from build123d import *

# Parameters (mm, degrees)
EXTRUDE_1_DEPTH          = 12
CUT_EXTRUDE_1_DEPTH      = 10
CUT_EXTRUDE_1_DEPTH_BACK = 10
SKETCH_2_W               = 2.506204129
SKETCH_2_H               = 10.984391515
EXTRUDE_START            = -1.5
EXTRUDE_2_DEPTH          = 1.5
FILLET_1_R               = 0.4
EXTRUDE_3_DEPTH          = 1.5
EXTRUDE_4_REACH          = 26.208


with BuildPart() as part:
    # 草图1 → 凸台-拉伸1 (new, symmetric)
    with BuildSketch(Plane(origin=(0, 0, 0), x_dir=(0, 0, -1), z_dir=(1, 0, 0))):
        with BuildLine():
            ThreePointArc((0.424459717, 1.438691749), (-1.23881175, -0.84578097), (1.494480371, -0.128562902))
            Line((1.494480371, -0.128562902), (0.897098533, 0.285679978))
            Line((0.897098533, 0.285679978), (0.611565164, 0.285679978))
            ThreePointArc((0.611565164, 0.285679978), (0.658950486, 0.146319025), (0.675, 0))
            ThreePointArc((0.675, 0), (-0.609153227, -0.290787458), (0.424459717, 0.524841832))
            Line((0.424459717, 0.524841832), (0.424459717, 1.438691749))
        make_face()
        with BuildLine():
            Line((8.48773274, -4.977898486), (8.91741162, -4.358256311))
            Line((8.91741162, -4.358256311), (0.854750449, 1.232640122))
            ThreePointArc((0.854750449, 1.232640122), (1.328932969, 0.695655923), (1.5, 0))
            ThreePointArc((1.5, 0), (1.498619458, -0.064340668), (1.494480371, -0.128562902))
            Line((1.494480371, -0.128562902), (8.48773274, -4.977898486))
        make_face()
        with BuildLine():
            ThreePointArc((1.5, 0), (1.328932969, 0.695655923), (0.854750449, 1.232640122))
            ThreePointArc((0.854750449, 1.232640122), (0.647849504, 1.352882485), (0.424459717, 1.438691749))
            Line((0.424459717, 1.438691749), (0.424459717, 0.524841832))
            ThreePointArc((0.424459717, 0.524841832), (0.531635671, 0.415918878), (0.611565164, 0.285679978))
            Line((0.611565164, 0.285679978), (0.897098533, 0.285679978))
            Line((0.897098533, 0.285679978), (1.494480371, -0.128562902))
            ThreePointArc((1.494480371, -0.128562902), (1.498619458, -0.064340668), (1.5, 0))
        make_face()
    extrude(amount=EXTRUDE_1_DEPTH, both=True)

    # 草图2 → 切除-拉伸1 (cut, two sides: drawn at the far end of the back side and taken through both)
    with BuildSketch(Plane(origin=(0, 0, 0), x_dir=(1, 0, 0), z_dir=(0, 1, 0)).offset(-CUT_EXTRUDE_1_DEPTH_BACK)):
        with Locations((-11.255680748, 7.657884592)):
            Rectangle(SKETCH_2_W, SKETCH_2_H)
        with Locations((11.255680748, 7.657884592)):
            Rectangle(SKETCH_2_W, SKETCH_2_H)
    extrude(amount=CUT_EXTRUDE_1_DEPTH + CUT_EXTRUDE_1_DEPTH_BACK, mode=Mode.SUBTRACT)

    # 草图3 → 凸台-拉伸2 (add)
    with BuildSketch(Plane.ZY.offset(12).offset(EXTRUDE_START)):
        with BuildLine():
            Line((1.209536672, 0.887142063), (4.315061937, -3.346956229))
            Line((4.315061937, -3.346956229), (2.791074167, -3.281580786))
            Line((2.791074167, -3.281580786), (-0.41583993, -1.441206839))
            ThreePointArc((-0.41583993, -1.441206839), (1.229955601, -0.858608886), (1.209536672, 0.887142063))
        make_face()
    extrude(amount=EXTRUDE_2_DEPTH)

    # 圆角1
    # the kernel refuses this fillet: 0.4 mm, written as the material it takes off along each edge
    with BuildSketch(Plane(origin=(0, -4.977898486, -8.48773274), x_dir=(0, 0.5698336328652603, 0.8217600810793743), z_dir=(-1, 0, 0)), Plane(origin=(0, -4.358256311, -8.91741162), x_dir=(0, 0.5698336328652598, 0.8217600810793746), z_dir=(1, 0, 0))) as fillet_1_piece_1:
        with BuildLine():
            CenterArc((FILLET_1_R, FILLET_1_R), FILLET_1_R, 180, 90)
            Line((0, FILLET_1_R), (0, 0))
            Line((0, 0), (FILLET_1_R, 0))
        make_face()
    extrude(amount=11.002578683, mode=Mode.SUBTRACT)
    with BuildSketch(Plane(origin=(0, -4.358256311, -8.91741162), x_dir=(0, 0.5698336328652598, 0.8217600810793746), z_dir=(-1, 0, 0)), Plane(origin=(0, -4.977898486, -8.48773274), x_dir=(0, 0.5698336328652603, 0.8217600810793743), z_dir=(1, 0, 0))) as fillet_1_piece_2:
        with BuildLine():
            CenterArc((FILLET_1_R, -FILLET_1_R), FILLET_1_R, 90, 90)
            Line((0, -FILLET_1_R), (0, 0))
            Line((0, 0), (FILLET_1_R, 0))
        make_face()
    extrude(amount=11.002578683, mode=Mode.SUBTRACT)

    # 草图4 → 凸台-拉伸3 (add)
    with BuildSketch(Plane(origin=(12, 0, 0), x_dir=(0, 0, -1), z_dir=(1, 0, 0))):
        with BuildLine():
            Line((-1.361590085, -0.629342864), (-0.064760058, -4.70678049))
            Line((-0.064760058, -4.70678049), (1.358347945, -5.014160577))
            Line((1.358347945, -5.014160577), (6.052641572, -4.70678049))
            Line((6.052641572, -4.70678049), (2.165688834, -0.593999427))
            Line((2.165688834, -0.593999427), (1.494480371, -0.128562902))
            ThreePointArc((1.494480371, -0.128562902), (0.259056171, -1.477460626), (-1.361590085, -0.629342864))
        make_face()
    extrude(amount=-EXTRUDE_3_DEPTH)

    # 凸台-拉伸4: up to this face of the body (flat: up to its plane)
    extrude_4_end = Plane(part.part.faces().sort_by_distance((12, -3.083366952, -2.010931635))[0])
    # 草图5 → 凸台-拉伸4 (add, up to the picked face)
    with BuildSketch(Plane(origin=(10.002578683, 0, 0), x_dir=(0, 0, -1), z_dir=(1, 0, 0)), mode=Mode.PRIVATE) as extrude_4_sk1:
        Polygon((6.052641572, -4.70678049), (2.165688834, -0.593999427), (2.165688834, 0.323595257), (7.146064321, -3.129949789), align=None)
    extrude_4_tool1 = split(extrude(extrude_4_sk1.sketch, amount=EXTRUDE_4_REACH, mode=Mode.PRIVATE), bisect_by=extrude_4_end, keep=Keep.BOTH, mode=Mode.PRIVATE)
    add(extrude_4_tool1.solids().sort_by(Axis((10.002579, -2.305975, -4.731819), (1, 0, 0)))[0])


solid = part.part
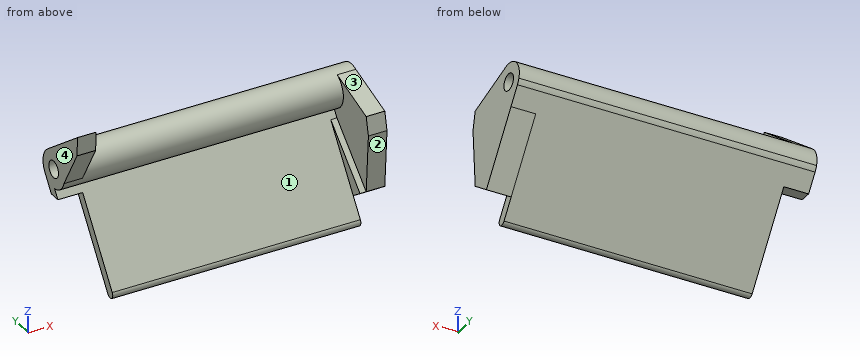
For this review, take the finished solid that the model builds, in its own axes (mm). Face numbers are marked on the shaded views. Round coordinates to 2 decimals unless told otherwise and drop trailing zeros. Write each loop counter-clockwise with the first axis right and the second up, starting at its lowest first coordinate (ties: lowest second). Pieces come first, ordered by that corner, then holes. Notation, with made-up numbers: (37.25, 0) -> (56.25, 0) arc R21 cw to (56.25, 23) -> close; hole circle Ø8 at (-11.5, -20.75). An arc over 180 degrees is marked (long way). Use CSV: the item, a comma, the result in double quotes.
(1) Consider section D-D, the plane z = -7.5. Give the boundary of the cut face in (x, y), plus the area to 3 significant figures.
Computed values:
outline,"(-10, -4.29) -> (10, -4.29) -> (10, -3.38) -> (-10, -3.38) -> close"
area,"18.4 mm²"
(2) To check wall thickness, follow L1, parallel to Y at x = 4, z = 0 (3 decimals); L2, parallel to Z at x = -9.75, y = -0.25; L3, parallel to X at y = -1.5, z = 0.5. State the ranges of each line that lie inside material, in increasing order. Write a range as [from, to].
Computed values:
L1,"[-1.5, -0.675], [0.675, 1.5]"
L2,"[-2.99, -1.67], [-1.48, -0.63], [0.63, 1.48]"
L3,"[-12, -10.5], [10.5, 12]"
(3) Consider section A-A, the plane y = -2. Give the boundary of the cut face in (x, z).
Computed values:
outline,"(-12, 0.56) -> (-10.5, 0.56) -> (-10.5, 3.33) -> (-12, 3.33) -> close; (-10, -5.52) -> (12, -5.52) -> (12, 0.93) -> (10.5, 0.93) -> (10.5, -3.49) -> (10, -3.49) -> (10, -4.19) -> (-10, -4.19) -> close"
(4) Consider section C-C, the plane z = 1.75. Give the boundary of the cut face in (x, y).
Computed values:
outline,"(-12, -2.68) -> (-10.5, -2.68) -> (-10.5, 0.15) -> (-12, 0.15) -> close"
(5) Clearance check with flat-ended pins moving along their axes: P1, Ø0.8, axis at y = -4, z = -7.5, coming from the +X side; P2, Ø3, axis at x = -4, z = -3, coming from the +Y side; P3, Ø1, axis at y = -3, z = -6, coming from the -X side; P4, Ø1.1, axis at y = 0, z = 0, coming from the -X side. State where each tip first meets the part, or that it passes through.
Computed values:
P1,"x = 10"
P2,"y = 0.79"
P3,"x = -10"
P4,"through"
(6) Draft analysis for pull direction Z (two halves, no side actions). For the marked faces 1, 2, 3 and 4, state which applies: +Z half, -Z half, draft (parallel to the pull), parting line (faces both ways), or undercut.
Computed values:
face 1,"undercut"
face 2,"-Z half"
face 3,"+Z half"
face 4,"draft"
(7) Consider section B-B, the plane x = -9.75. Give the boundary of the cut face in (y, z) (3 decimals), plus the area to 3 significant figures.
Computed values:
outline,"(-4.75, -8.159) arc R0.4 ccw to (-4.668, -8.702) arc R0.4 ccw to (-4.13, -8.589) -> (1.233, -0.855) arc R1.5 ccw (long way) to (-0.129, -1.494) -> close; hole circle Ø1.35 at (0, 0)"
area,"12.3 mm²"
